CAD build for the part. Positions are in the model's coordinates, mm. Face numbers are marked on the shaded views. A direction names the side the tool comes from. Give positions to 0.01 mm unless a question says otherwise; leave off trailing zeros. Loops run counter-clockwise (first coordinate to the right, second up) from the corner with the lowest first, then second, coordinate; pieces in that order, holes last. Notation, with made-up numbers: M 27.25,-4.5 L 32.25,-4.5 A25 ccw 32.25,29.5 Z; hole C 18.5,39 d6. An arc over 180 degrees is marked long. One line per question, with ' | ' between items.
```python
from build123d import *

# Parameters (mm, degrees)
F1_DEPTH       = 25
F3_D           = 3.75
F3_DEPTH       = 6
F3_CSINK_D     = 6.5
F3_CSINK_ANGLE = 70
F5_D           = 3.75
F5_DEPTH       = 6
F5_CSINK_D     = 6.5
F5_CSINK_ANGLE = 70


with BuildPart() as f1:
    # F0 (on Top) → F1 (new body)
    with BuildSketch(Plane.XY):
        Polygon((-23.20677, 6.948909), (-26.20677, 6.948909), (-26.20677, -6.051091), (37.79323, -6.051091), (37.79323, 6.948909), (34.79323, 6.948909), (34.79323, -5.051091), (-23.20677, -5.051091), align=None)
    extrude(amount=F1_DEPTH)

    # F3
    with Locations(Plane(origin=(-26.20677, 0, 0), x_dir=(0, -1, 0), z_dir=(-1, 0, 0))):
        with Locations((-1.448909, 12.5)):
            CounterSinkHole(F3_D / 2, F3_CSINK_D / 2, depth=F3_DEPTH, counter_sink_angle=F3_CSINK_ANGLE)

    # F5
    with Locations(Plane.YZ.offset(37.79323)):
        with Locations((1.448909, 12.5)):
            CounterSinkHole(F5_D / 2, F5_CSINK_D / 2, depth=F5_DEPTH, counter_sink_angle=F5_CSINK_ANGLE)


solid = f1.part
```
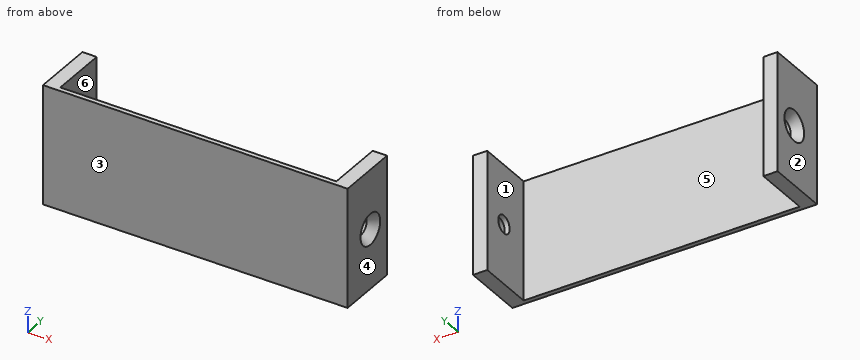
Item 1: 3-axis set-ups, long thin cutter, end or side, ignore diameter. For the marked faces 1 and 2: which of +Z, -Z, +X, -X, +Y, -Y reach the whole face in a straight line?
Conclusion:
face 1: +Z, -Z, +Y | face 2: +Z, -Z, -X, +Y, -Y
Item 2: Saw through at B-B on z = 12.5. Give the cut face in (x, y).
Conclusion:
outline: M -26.21,-6.05 L 37.79,-6.05 L 37.79,-1.8 L 35.83,-0.43 L 34.79,-0.43 L 34.79,-5.05 L -23.21,-5.05 L -23.21,-0.43 L -24.24,-0.43 L -26.21,-1.8 Z; M -26.21,4.7 L -24.24,3.32 L -23.21,3.32 L -23.21,6.95 L -26.21,6.95 Z; M 34.79,3.32 L 35.83,3.32 L 37.79,4.7 L 37.79,6.95 L 34.79,6.95 Z
Item 3: Saw through at C-C on z = 23. Give the cut face in (x, y).
Conclusion:
outline: M -26.21,-6.05 L 37.79,-6.05 L 37.79,6.95 L 34.79,6.95 L 34.79,-5.05 L -23.21,-5.05 L -23.21,6.95 L -26.21,6.95 Z
Item 4: Drill centre lines: line 1 along X through (y, z) = (0.75, 3.5); line 2 along Y through (x, z) = (35.2, 12.5); line 3 along Y through (x, z) = (-4.5, 14.75). Where is each one in solid material? Low to high. Write a range as [from, to].
Conclusion:
line 1: [-26.21, -23.21], [34.79, 37.79] | line 2: [-6.05, -0.43], [3.32, 6.95] | line 3: [-6.05, -5.05]
Item 5: Mould opens along X. For the marked faces 3, 4, 5 and 6 say: pulls with the +X half, pulls with the -X half, needs draft (parallel to the pull), parting line crosses it, or undercut.
Conclusion:
face 3: needs draft | face 4: pulls with the +X half | face 5: undercut | face 6: undercut
Item 6: Saw through at D-D on x = 24.5. Give the cut face in (y, z).
Conclusion:
outline: M -6.05,0 L -5.05,0 L -5.05,25 L -6.05,25 Z
Item 7: Saw through at A-A on y = -3.5. Give the cut face in (x, z).
Conclusion:
outline: M -26.21,0 L -23.21,0 L -23.21,25 L -26.21,25 Z; M 34.79,0 L 37.79,0 L 37.79,25 L 34.79,25 Z
Item 8: Drop flat-ended pins along their axis: P1, Ø6, axis at y = 1.45, z = 12.5, coming from the +X side; P2, Ø2, axis at y = 1.45, z = 12.5, coming from the +X side; P3, Ø1, axis at x = -4.5, z = 5.5, coming from the +Y side. Give the stop position or say it passes through.
Conclusion:
P1: x = 37.44 | P2: through | P3: y = -5.05
